Design review of the part built by this model. Coordinates are the model's own, in mm. A direction names the side the tool comes from. Round coordinates to 2 decimals unless told otherwise and drop trailing zeros. Loops run counter-clockwise (first coordinate to the right, second up) from the corner with the lowest first, then second, coordinate; pieces in that order, holes last. Notation, with made-up numbers: (11.5, 12) -> (42.5, 12) arc R8 cw to (42.5, 27) -> close; hole circle Ø3 at (12.5, 5). An arc over 180 degrees is marked (long way). Use a Markdown table: item, result. Add a question column.
from build123d import *

# Parameters (mm, degrees)
SKETCH_1_W               = 400
SKETCH_1_H               = 400
EXTRUDE_1_DEPTH          = 16
SKETCH_2_W               = 16
SKETCH_2_H               = 370
EXTRUDE_2_DEPTH          = 400
SKETCH_3_W               = 16
SKETCH_3_H               = 370
EXTRUDE_3_DEPTH          = 400
SKETCH_4_W               = 368
SKETCH_4_H               = 16
EXTRUDE_4_DEPTH          = 340
EXTRUDE_5_REACH          = 687.53
SKETCH_6_W               = 305
SKETCH_6_H               = 16
SKETCH_7_W               = 22
SKETCH_7_H               = 16
CUT_EXTRUDE_1_DEPTH      = 5
SKETCH_14_W              = 22
SKETCH_14_H              = 16
CUT_EXTRUDE_2_DEPTH      = 5
SKETCH_15_W              = 1.5
SKETCH_15_H              = 2.5
CUT_EXTRUDE_3_DEPTH      = 25
MIRROR_4_COPY_1_SKETCH_W = 1.5
MIRROR_4_COPY_1_SKETCH_H = 2.5
MIRROR_4_COPY_1_DEPTH    = 25
MIRROR_4_COPY_2_SKETCH_W = 1.5
MIRROR_4_COPY_2_SKETCH_H = 2.5
MIRROR_4_COPY_2_DEPTH    = 25
MIRROR_4_COPY_3_SKETCH_W = 1.5
MIRROR_4_COPY_3_SKETCH_H = 2.5
MIRROR_4_COPY_3_DEPTH    = 25
MIRROR_4_COPY_4_SKETCH_W = 1.5
MIRROR_4_COPY_4_SKETCH_H = 2.5
MIRROR_4_COPY_4_DEPTH    = 25


with BuildPart() as part:
    # 草图1 → 凸台-拉伸1 (new body)
    with BuildSketch(Plane.XY):
        with Locations((186.413251901, 186.573625287)):
            Rectangle(SKETCH_1_W, SKETCH_1_H)
    extrude(amount=EXTRUDE_1_DEPTH)

    # 草图2 → 凸台-拉伸2 (add)
    with BuildSketch(Plane.XY.offset(16)):
        with Locations((-5.586748099, 201.573625287)):
            Rectangle(SKETCH_2_W, SKETCH_2_H)
    extrude(amount=EXTRUDE_2_DEPTH)

    # 草图3 → 凸台-拉伸3 (add)
    with BuildSketch(Plane.XY.offset(16)):
        with Locations((378.413251901, 201.573625287)):
            Rectangle(SKETCH_3_W, SKETCH_3_H)
    extrude(amount=EXTRUDE_3_DEPTH)

    # 草图4 → 凸台-拉伸4 (add)
    with BuildSketch(Plane.XY.offset(16)):
        with Locations((186.413251901, 378.573625287)):
            Rectangle(SKETCH_4_W, SKETCH_4_H)
    extrude(amount=EXTRUDE_4_DEPTH)

    # 草图6 → 凸台-拉伸5 (add, up to next)
    with BuildSketch(Plane.ZY.offset(-370.413251901), mode=Mode.PRIVATE) as extrude_5_sk1:
        with Locations((203.5, 24.573625287)):
            Rectangle(SKETCH_6_W, SKETCH_6_H)
    extrude_5_tool1 = extrude(extrude_5_sk1.sketch, amount=EXTRUDE_5_REACH, mode=Mode.PRIVATE) - part.part
    add(extrude_5_tool1.solids().sort_by_distance((370.413252, 24.573625, 203.5))[0])

    # 草图7 → 切除-拉伸1 (cut)
    with BuildSketch(Plane.XY.offset(356)):
        with Locations((359.413251901, 24.573625287)):
            Rectangle(SKETCH_7_W, SKETCH_7_H)
    cut_extrude_1 = extrude(amount=-CUT_EXTRUDE_1_DEPTH, mode=Mode.SUBTRACT)

    # 草图14 → 切除-拉伸2 (cut)
    with BuildSketch(Plane.XY.offset(356)):
        with Locations((13.413251901, 24.573625287)):
            Rectangle(SKETCH_14_W, SKETCH_14_H)
    cut_extrude_2 = extrude(amount=-CUT_EXTRUDE_2_DEPTH, mode=Mode.SUBTRACT)

    # 镜向1: 切除-拉伸1, 切除-拉伸2 across plane
    add(cut_extrude_1.mirror(Plane(origin=(0, 201.573625287, 0), x_dir=(0, 0, 1), z_dir=(0, -1, 0))), mode=Mode.SUBTRACT)
    add(cut_extrude_2.mirror(Plane(origin=(0, 201.573625287, 0), x_dir=(0, 0, 1), z_dir=(0, -1, 0))), mode=Mode.SUBTRACT)

    # 草图15 → 切除-拉伸3 (cut)
    with BuildSketch(Plane.XZ.offset(-16.573625287)):
        with Locations((1.663251901, 357.25)):
            Rectangle(SKETCH_15_W, SKETCH_15_H)
    cut_extrude_3 = extrude(amount=-CUT_EXTRUDE_3_DEPTH, mode=Mode.SUBTRACT)

    # 镜向2: 切除-拉伸3 across plane
    add(cut_extrude_3.mirror(Plane(origin=(0, 201.573625287, 0), x_dir=(0, 0, 1), z_dir=(0, -1, 0))), mode=Mode.SUBTRACT)

    # 镜向3: 切除-拉伸3 across plane
    add(cut_extrude_3.mirror(Plane(origin=(186.413251901, 0, 0), x_dir=(0, 0, 1), z_dir=(1, 0, 0))), mode=Mode.SUBTRACT)

    # 镜向4 copy 1 sketch → 镜向4 copy 1 (cut)
    with BuildSketch(Plane.XZ.offset(-16.573625287)):
        with Locations((1.663251901, 357.25)):
            Rectangle(MIRROR_4_COPY_1_SKETCH_W, MIRROR_4_COPY_1_SKETCH_H)
    extrude(amount=-MIRROR_4_COPY_1_DEPTH, mode=Mode.SUBTRACT)

    # 镜向4 copy 2 sketch → 镜向4 copy 2 (cut)
    with BuildSketch(Plane(origin=(0, 386.573625287, 0), x_dir=(1, 0, 0), z_dir=(0, 1, 0))):
        with Locations((1.663251901, -357.25)):
            Rectangle(MIRROR_4_COPY_2_SKETCH_W, MIRROR_4_COPY_2_SKETCH_H)
    extrude(amount=-MIRROR_4_COPY_2_DEPTH, mode=Mode.SUBTRACT)

    # 镜向4 copy 3 sketch → 镜向4 copy 3 (cut)
    with BuildSketch(Plane(origin=(372.826503801, 386.573625287, 0), x_dir=(-1, 0, 0), z_dir=(0, 1, 0))):
        with Locations((1.663251901, 357.25)):
            Rectangle(MIRROR_4_COPY_3_SKETCH_W, MIRROR_4_COPY_3_SKETCH_H)
    extrude(amount=-MIRROR_4_COPY_3_DEPTH, mode=Mode.SUBTRACT)

    # 镜向4 copy 4 sketch → 镜向4 copy 4 (cut)
    with BuildSketch(Plane(origin=(0, 386.573625287, 0), x_dir=(1, 0, 0), z_dir=(0, 1, 0))):
        with Locations((1.663251901, -357.25)):
            Rectangle(MIRROR_4_COPY_4_SKETCH_W, MIRROR_4_COPY_4_SKETCH_H)
    extrude(amount=-MIRROR_4_COPY_4_DEPTH, mode=Mode.SUBTRACT)


solid = part.part
1. Mouldability with a two-part tool opening along Y and no side actions: class faces 1 (the face through (184, 370.574, 184)), 2 (the face through (13, 378, 351)), 3 (the face through (184, -13.426, 8)) as +Y half, -Y half, draft (parallel to the pull), parting line (faces both ways), or undercut.
2. For faces 4 (the face through (189, 32.574, 201)), 5 (the face through (386.413, 184, 205)), 6 (the face through (184, 16.574, 213)), 7 (the face through (189, 24, 51)), 8 (the face through (359, 378, 351)), list the 3-axis set-ups (+Z, -Z, +X, -X, +Y, -Y) from which the entire face can be reached by the end or side of a thin tool; tool diameter is ignored.
3. Consider section A-A on z = 385. State the section outline as (x, y) points, plus the area to 3 significant figures.
4. To check wall thickness, follow probe 1 along X at (y, z) = (126.5, 316.5); probe 2 along Y at (x, z) = (138, 132.5); probe 3 along Z at (x, y) = (197.5, 311). State the ranges of each line that lie inside material, in increasing order. Write a range as from..to.
5. Consider section D-D on y = 138.5. State the section outline as (x, z) points.
6. Consider section B-B on x = 96.5. State the section outline as (y, z) points.
7. Insertion check: P1, Ø0.8, axis at x = 371, z = 357, coming from the -Y side; P2, Ø5, axis at x = 356, y = 382.5, coming from the +Z side; P3, Ø13, axis at x = 237, y = 21.5, coming from the +Z side. Each pin has a flat end and moves straight along its axis. Give the tip position at first contact, or say it passes through.
8. Consider section C-C on z = 166. State the section outline as (x, y) points.
Verdict:
| question | item | result |
|---|---|---|
| 1 | face 1 | undercut |
| 1 | face 2 | draft |
| 1 | face 3 | -Y half |
| 2 | face 4 | +Z |
| 2 | face 5 | +Z, -Z, +X, +Y, -Y |
| 2 | face 6 | +Z, +X, -X, -Y |
| 2 | face 7 | -Y |
| 2 | face 8 | +Z, +Y, -Y |
| 3 | outline | (-13.59, 16.57) -> (2.41, 16.57) -> (2.41, 386.57) -> (-13.59, 386.57) -> close; (370.41, 16.57) -> (386.41, 16.57) -> (386.41, 386.57) -> (370.41, 386.57) -> close |
| 3 | area | 11,800 mm² |
| 4 | probe 1 | x = -13.59..2.41, 370.41..386.41 |
| 4 | probe 2 | y = 16.57..32.57, 370.57..386.57 |
| 4 | probe 3 | z = 0..16 |
| 5 | outline | (-13.59, 0) -> (386.41, 0) -> (386.41, 416) -> (370.41, 416) -> (370.41, 16) -> (2.41, 16) -> (2.41, 416) -> (-13.59, 416) -> close |
| 6 | outline | (-13.43, 0) -> (386.57, 0) -> (386.57, 356) -> (370.57, 356) -> (370.57, 16) -> (-13.43, 16) -> close; (16.57, 51) -> (32.57, 51) -> (32.57, 356) -> (16.57, 356) -> close |
| 7 | P1 | stops at y = 41.57 |
| 7 | P2 | stops at z = 351 |
| 7 | P3 | stops at z = 356 |
| 8 | outline | (-13.59, 16.57) -> (386.41, 16.57) -> (386.41, 386.57) -> (-13.59, 386.57) -> close; hole (2.41, 32.57) -> (370.41, 32.57) -> (370.41, 370.57) -> (2.41, 370.57) -> close |
